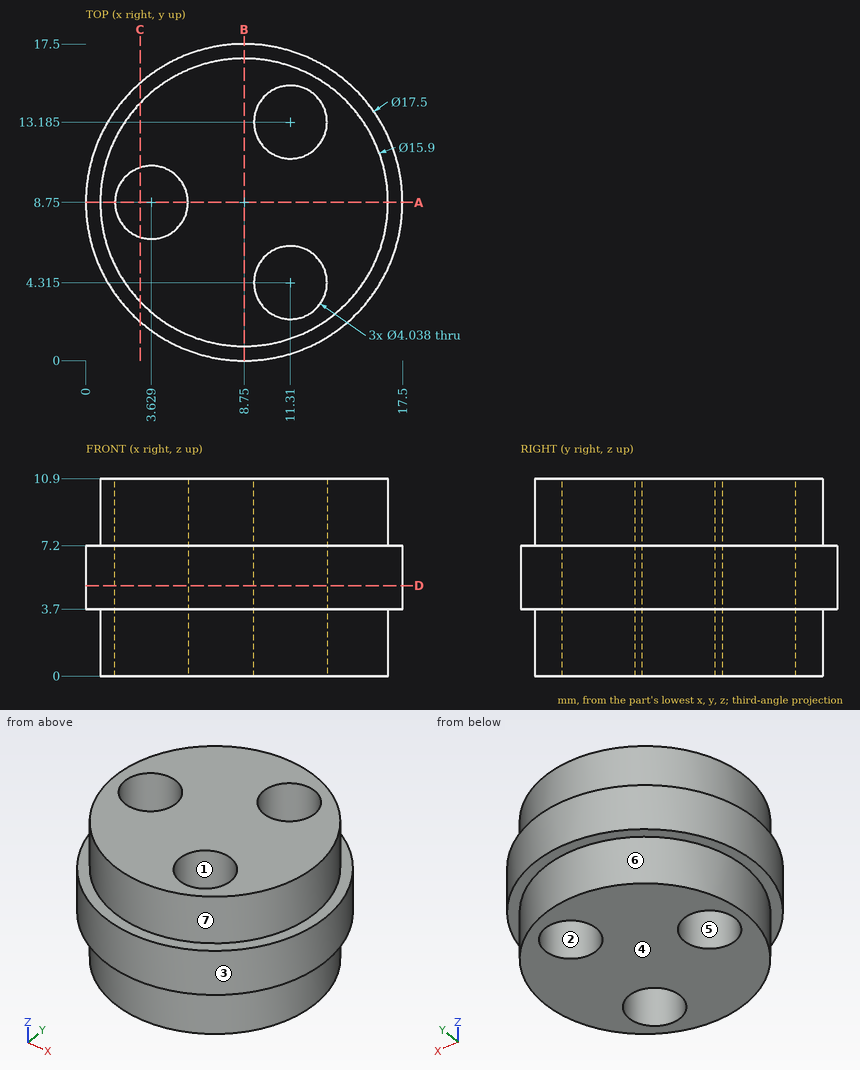
Answer from the drawing. Dimensions are ordinates in mm from the lowest x, y and z of the part. A direction names the side the tool comes from. Round coordinates to 2 decimals unless told otherwise and drop trailing zeros. Order: outer loops, then holes, each group sorted by start corner. A loop starts at its lowest first (then second) coordinate and runs counter-clockwise, first axis right, second up. Notation, with made-up numbers: (-21.75, 58) - (3.25, 58) arc R23 cw to (3.25, 70) - close; hole circle Ø2 at (33.5, 3). An arc over 180 degrees is marked (long way). Put each result on its own line as item: value. Start each with the question number.
(1) Find section A-A (y = 8.75). Give the vertices of the cut face in (x, z), plus the area to 3 significant figures.
(2) Determine the mould class of the marked faces 1, 2, 3 and 4 for opening direction X: released by +X, released by -X, zero draft, split by the parting line, or undercut.
(3) Find section B-B (x = 8.75). Give the vertices of the cut face in (y, z), plus the area to 3 significant figures.
(4) Straight lines are drawn through the part: probe 1 along Y at (x, z) = (13, 8.5); probe 2 along Y at (x, z) = (12, 7.25) (1 decimal); probe 3 along Y at (x, z) = (3, 3.75) (1 decimal). For each, find the intervals that lie inside material, in ascending order. Write a range as from..to.
(5) Find section D-D (z = 5). State how many separate pieces and enclosed holes the cut face has, plus the area to 3 significant figures.
(6) Find section C-C (x = 3). Give the vertices of the cut face in (y, z) (1 decimal), plus the area to 3 significant figures.
(7) For the marked faces 5, 6 and 7, determine the directions among +Z, -Z, +X, -X, +Y, -Y from which every point of the face is accessible in a straight line to the end or side of a thin tool.
Reply:
1. outline: (0, 3.7) - (0.8, 3.7) - (0.8, 0) - (1.61, 0) - (1.61, 10.9) - (0.8, 10.9) - (0.8, 7.2) - (0, 7.2) - close; (5.65, 0) - (16.7, 0) - (16.7, 3.7) - (17.5, 3.7) - (17.5, 7.2) - (16.7, 7.2) - (16.7, 10.9) - (5.65, 10.9) - close
1. area: 135 mm^2
2. face 1: undercut
2. face 2: undercut
2. face 3: split by the parting line
2. face 4: zero draft
3. outline: (0, 3.7) - (0.8, 3.7) - (0.8, 0) - (16.7, 0) - (16.7, 3.7) - (17.5, 3.7) - (17.5, 7.2) - (16.7, 7.2) - (16.7, 10.9) - (0.8, 10.9) - (0.8, 7.2) - (0, 7.2) - close
3. area: 179 mm^2
4. probe 1: 2.03..3.21, 5.42..12.08, 14.29..15.47
4. probe 2: 1.5..2.4, 6.2..11.3, 15.1..16
4. probe 3: 2.2..6.8, 10.7..15.3
5. separate pieces: 1
5. enclosed holes: 3
5. area: 202 mm^2
6. outline: (2.2, 3.7) - (3.3, 3.7) - (3.3, 0) - (6.8, 0) - (6.8, 10.9) - (3.3, 10.9) - (3.3, 7.2) - (2.2, 7.2) - close; (10.7, 0) - (14.2, 0) - (14.2, 3.7) - (15.3, 3.7) - (15.3, 7.2) - (14.2, 7.2) - (14.2, 10.9) - (10.7, 10.9) - close
6. area: 85.6 mm^2
7. face 5: +Z, -Z
7. face 6: -Z
7. face 7: +Z
